Geometry: final body of the model. Coordinates: model frame, mm. Give positions to 0.01 mm unless a question says otherwise; leave off trailing zeros. Write each loop counter-clockwise with the first axis right and the second up, starting at its lowest first coordinate (ties: lowest second). Pieces come first, ordered by that corner, then holes.
Q1. Section A-A (x = 0). Return the cut outline in (y, z).
Q2. Section C-C (y = -6). State how many separate pieces and enclosed holes the cut face has, plus the area to 3 significant figures.
Q3. Section B-B (z = -298.45). Return the cut outline in (x, y).
Q4. Line query: line 1 (Z direction, x = 0, y = -4.75); line 2 (Z direction, x = -13, y = -8); line 3 (X direction, y = -2.75, z = -286.5). Output: solid intervals per line, ascending.
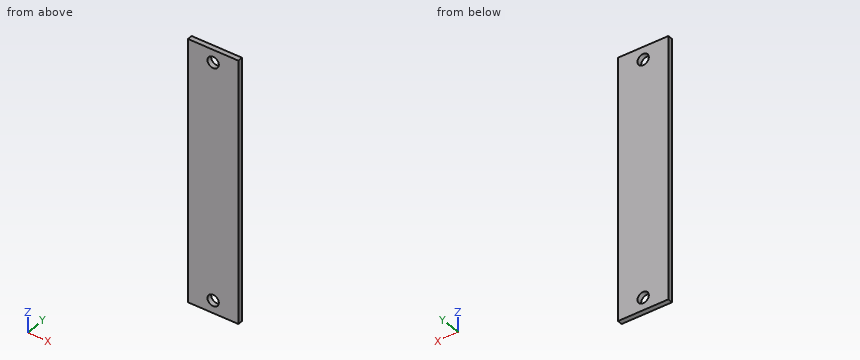
from build123d import *

# Parameters (mm, degrees)
F0_W     = 127
F0_H     = 660.4
F0_R     = 14.2875
F1_DEPTH = 9.525
F2_DEPTH = 12.7


with BuildPart() as f1:
    # F0 (on Front) → F1 (new body)
    with BuildSketch(Plane.XZ):
        Rectangle(F0_W, F0_H)
        with Locations((0, -298.45)):
            Circle(F0_R, mode=Mode.SUBTRACT)
        with Locations((0, 298.45)):
            Circle(F0_R, mode=Mode.SUBTRACT)
    extrude(amount=F1_DEPTH)

    # F0 (on Front) → F2 (join)
    with BuildSketch(Plane.XZ):
        Rectangle(F0_W, F0_H)
        with Locations((0, -298.45)):
            Circle(F0_R, mode=Mode.SUBTRACT)
        with Locations((0, 298.45)):
            Circle(F0_R, mode=Mode.SUBTRACT)
    extrude(amount=F2_DEPTH)


solid = f1.part
Computed:
1. outline: (-12.7, -330.2) - (0, -330.2) - (0, -312.74) - (-12.7, -312.74) - close; (-12.7, -284.16) - (0, -284.16) - (0, 284.16) - (-12.7, 284.16) - close; (-12.7, 312.74) - (0, 312.74) - (0, 330.2) - (-12.7, 330.2) - close
2. separate pieces: 1
2. enclosed holes: 2
2. area: 82,600 mm2
3. outline: (-63.5, -12.7) - (-14.29, -12.7) - (-14.29, 0) - (-63.5, 0) - close; (14.29, -12.7) - (63.5, -12.7) - (63.5, 0) - (14.29, 0) - close
4. line 1: z = -330.2 to -312.74, -284.16 to 284.16, 312.74 to 330.2
4. line 2: z = -330.2 to -304.38, -292.52 to 292.52, 304.38 to 330.2
4. line 3: x = -63.5 to -7.83, 7.83 to 63.5
